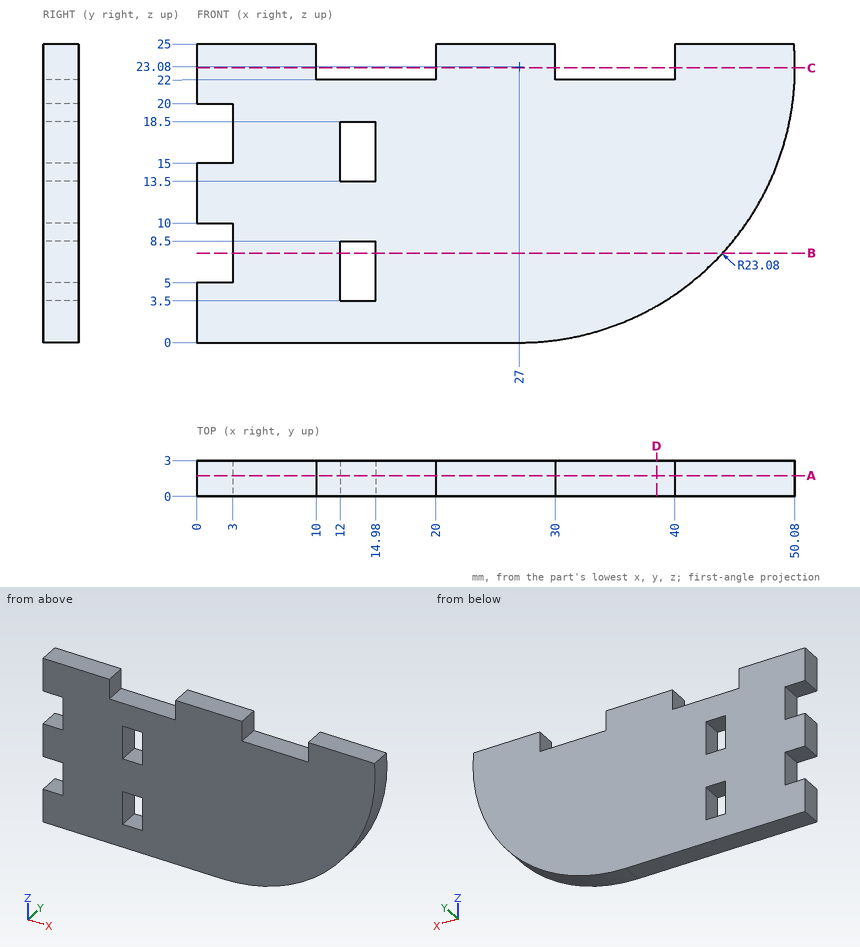
Here's the drawing with two shaded views (mm, measured from the low corner). I have some questions. Give positions to 0.01 mm unless a question says otherwise; leave off trailing zeros. Write each loop counter-clockwise with the first axis right and the second up, starting at its lowest first coordinate (ties: lowest second). Pieces come first, ordered by that corner, then holes. Notation, with made-up numbers: (23.25, 52) -> (56.25, 52) arc R22 cw to (56.25, 88) -> close; hole circle Ø3 at (31.25, 60.5). An arc over 180 degrees is marked (long way). Answer as a JSON object with one key per item and string values. Group by question number.
Item 1: Suppose I cut it at B-B (z = 7.5). Please give me the cut outline in (x, y), plus the area to 3 significant figures.
Item 2: Please list where these lines run through material, in increasing order: line 1 (Z direction, x = 14, y = 0.85); line 2 (X direction, y = 2.8, z = 23.25); line 3 (X direction, y = 1.5, z = 7). Write a range as [from, to].
Item 3: Suppose I cut it at D-D (x = 38.5). Please give me the cut outline in (y, z), plus the area to 3 significant figures.
Item 4: I'm going to push flat-ended pins straight in: P1, Ø1, axis at x = 35.5, y = 0.5, coming from the +Z side; P2, Ø6, axis at x = 31, z = 9, coming from the -Y side. Where does each tip first touch, or does it pass through?
Item 5: Suppose I cut it at C-C (z = 23). Please give me the cut outline in (x, y), plus the area to 3 significant figures.
Item 6: Suppose I cut it at A-A (y = 1.75). Please give me the cut outline in (x, z), plus the area to 3 significant figures.
Findings:
{
 "1": {"outline": "(3, 0) -> (12, 0) -> (12, 3) -> (3, 3) -> close; (14.98, 0) -> (44.03, 0) -> (44.03, 3) -> (14.98, 3) -> close", "area": "114 mm²"},
 "2": {"line 1": "z = [0, 3.5], [8.5, 13.5], [18.5, 22]", "line 2": "x = [0, 10], [20, 30], [40, 50.08]", "line 3": "x = [3, 12], [14.98, 43.56]"},
 "3": {"outline": "(0, 3.07) -> (3, 3.07) -> (3, 22) -> (0, 22) -> close", "area": "56.8 mm²"},
 "4": {"P1": "stops at z = 22", "P2": "stops at y = 0"},
 "5": {"outline": "(0, 0) -> (10, 0) -> (10, 3) -> (0, 3) -> close; (20, 0) -> (30, 0) -> (30, 3) -> (20, 3) -> close; (40, 0) -> (50.08, 0) -> (50.08, 3) -> (40, 3) -> close", "area": "90.2 mm²"},
 "6": {"outline": "(0, 0) -> (27, 0) arc R23.08 ccw to (50, 25) -> (40, 25) -> (40, 22) -> (30, 22) -> (30, 25) -> (20, 25) -> (20, 22) -> (10, 22) -> (10, 25) -> (0, 25) -> (0, 20) -> (3, 20) -> (3, 15) -> (0, 15) -> (0, 10) -> (3, 10) -> (3, 5) -> (0, 5) -> close; hole (12, 3.5) -> (14.98, 3.5) -> (14.98, 8.5) -> (12, 8.5) -> close; hole (12, 13.5) -> (14.98, 13.5) -> (14.98, 18.5) -> (12, 18.5) -> close", "area": "1,020 mm²"}
}
